```python
from build123d import *

# Parameters (mm, degrees)
SKETCH1_R                          = 12.2
BOSS_EXTRUDE1_DEPTH                = 12.3
SKETCH2_R                          = 3.225
BOSS_EXTRUDE2_DEPTH                = 1
SKETCH3_R                          = 3.05
BOSS_EXTRUDE3_DEPTH                = 0.5
SKETCH4_R                          = 1
BOSS_EXTRUDE4_DEPTH                = 5.95
FILLET1_R                          = 1
FILLET2_R                          = 0.5
TAP_DRILL_FOR_M1_6X0_35_TAP1_D     = 1.25
TAP_DRILL_FOR_M1_6X0_35_TAP1_DEPTH = 1.1
TAP_DRILL_FOR_M1_6X0_35_TAP1_TIP   = 0.375537887
CUT_EXTRUDE1_START                 = -0.5
SKETCH8_R                          = 11.7
SKETCH8_R_2                        = 3.05
CUT_EXTRUDE1_DEPTH                 = 0.5


with BuildPart() as part:
    # Sketch1 → Boss-Extrude1 (new body)
    with BuildSketch(Plane(origin=(0, 0, 0), x_dir=(1, 0, 0), z_dir=(0, 1, 0))):
        with Locations(Location((0, 0, 0), (0, 0, 270))):
            Circle(SKETCH1_R)
    extrude(amount=BOSS_EXTRUDE1_DEPTH)

    # Sketch2 → Boss-Extrude2 (add)
    with BuildSketch(Plane(origin=(0, 12.3, 0), x_dir=(1, 0, 0), z_dir=(0, 1, 0))):
        with Locations(Location((0, 0, 0), (0, 0, 270))):
            Circle(SKETCH2_R)
    extrude(amount=BOSS_EXTRUDE2_DEPTH)

    # Sketch3 → Boss-Extrude3 (add)
    with BuildSketch(Plane.XZ):
        with Locations(Location((0, 0, 0), (0, 0, 90))):
            Circle(SKETCH3_R)
    extrude(amount=BOSS_EXTRUDE3_DEPTH)

    # Sketch4 → Boss-Extrude4 (add)
    with BuildSketch(Plane(origin=(0, 13.3, 0), x_dir=(1, 0, 0), z_dir=(0, 1, 0))):
        with Locations(Location((0, 0, 0), (0, 0, 270))):
            Circle(SKETCH4_R)
    extrude(amount=BOSS_EXTRUDE4_DEPTH)

    # Fillet1
    fillet1_edges = [part.edges().sort_by_distance(p)[0] for p in [
        (0, 12.3, -12.2),
    ]]
    fillet(fillet1_edges, radius=FILLET1_R)

    # Fillet2
    fillet2_edges = [part.edges().sort_by_distance(p)[0] for p in [
        (0, 19.25, -1),
        (0, 13.3, -3.225),
    ]]
    fillet(fillet2_edges, radius=FILLET2_R)

    # Tap Drill for M1.6x0.35 Tap1
    with Locations(Plane(origin=(0, 12.3, 0), x_dir=(1, 0, 0), z_dir=(0, 1, 0))):
        with Locations((0, -8.25), (-7.144709581, -4.125), (-7.144709581, 4.125), (0, 8.25), (7.144709581, 4.125), (7.144709581, -4.125)):
            Hole(TAP_DRILL_FOR_M1_6X0_35_TAP1_D / 2, depth=TAP_DRILL_FOR_M1_6X0_35_TAP1_DEPTH)
            with Locations((0, 0, -(TAP_DRILL_FOR_M1_6X0_35_TAP1_DEPTH + TAP_DRILL_FOR_M1_6X0_35_TAP1_TIP / 2))):  # 118° drill point
                Cone(0, TAP_DRILL_FOR_M1_6X0_35_TAP1_D / 2, TAP_DRILL_FOR_M1_6X0_35_TAP1_TIP, mode=Mode.SUBTRACT)

    # Sketch8 → Cut-Extrude1 (cut)
    with BuildSketch(Plane.XZ.offset(CUT_EXTRUDE1_START)):
        with Locations(Location((0, 0, 0), (0, 0, 270))):
            Circle(SKETCH8_R)
        with Locations(Location((0, 0, 0), (0, 0, 270))):
            Circle(SKETCH8_R_2, mode=Mode.SUBTRACT)
    extrude(amount=CUT_EXTRUDE1_DEPTH, mode=Mode.SUBTRACT)


solid = part.part
```
The model under review builds one solid part; all positions refer to its coordinate system, in mm. A direction names the side the tool comes from. Round coordinates to 2 decimals unless told otherwise and drop trailing zeros. Loops run counter-clockwise (first coordinate to the right, second up) from the corner with the lowest first, then second, coordinate; pieces in that order, holes last. Notation, with made-up numbers: (-2, 5) -> (12, 5) arc R13 cw to (12, 18) -> close; hole circle Ø2 at (35.25, 0.5). An arc over 180 degrees is marked (long way). Answer in a Markdown table with one row per item.
1) Consider section B-B, the plane y = 6.5. Write out the cut boundary in (x, z).
Taken from the geometry:
| item | result |
|---|---|
| outline | circle Ø24.4 at (0, 0) |
2) Tool access review of faces 4 (the cylindrical face through (-7.722, 11.742, 4.364)), 5 (the flat face through (0, -0.5, 0)), 6 (the cylindrical face through (-10.38, 0.25, -5.4)): name each direction out of +Z, -Z, +X, -X, +Y, -Y from which nothing blocks a thin tool from reaching the whole face with its end or side.
Taken from the geometry:
| item | result |
|---|---|
| face 4 | +Y |
| face 5 | +Z, -Z, +X, -X, -Y |
| face 6 | -Y |
3) For pin 1 Ø10 at (x, y) = (6, 14) entering from +Z; pin 2 Ø12 at (x, z) = (-9, -9) entering from +Y; pin 3 Ø1.4 at (x, z) = (7.14, 4.12) entering from -Y, all flat-tipped, find the tip position at first contact; note any pin that passes through.
Taken from the geometry:
| item | result |
|---|---|
| pin 1 | stops at z = 12.07 |
| pin 2 | stops at y = 12.3 |
| pin 3 | stops at y = 0.5 |
4) Consider section A-A, the plane y = 17.75. Write out the cut boundary in (x, z), plus the area to 3 significant figures.
Taken from the geometry:
| item | result |
|---|---|
| outline | circle Ø2 at (0, 0) |
| area | 3.14 mm² |
5) Draft analysis for pull direction Z (two halves, no side actions). For faces 1 (the flat face through (3, 12.3, 2)), 2 (the cylindrical face through (-7.74, 11.74, -4.31)), 3 (the cylindrical face through (-1, 16, 0)), state which applies: pulls with the +Z half, pulls with the -Z half, needs draft (parallel to the pull), parting line crosses it, or undercut.
Taken from the geometry:
| item | result |
|---|---|
| face 1 | needs draft |
| face 2 | undercut |
| face 3 | parting line crosses it |
6) Wall thickness on line 1 along X through (y, z) = (0.25, 0); line 2 along Y through (x, z) = (-9.75, -1.25); line 3 along Y through (x, z) = (2, 0): over which ranges is each line inside the solid? List them lowest first.
Taken from the geometry:
| item | result |
|---|---|
| line 1 | x = -12.2 to -11.7, -3.05 to 3.05, 11.7 to 12.2 |
| line 2 | y = 0.5 to 12.3 |
| line 3 | y = -0.5 to 13.3 |
